Autodesk Inventor part; units mm, degrees
ref_plane "YZ Plane" through (0, 0, 0) normal (1, 0, 0) x (0, 1, 0)
ref_plane "XZ Plane" through (0, 0, 0) normal (0, 1, 0) x (-1, 0, 0)
ref_plane "XY Plane" through (0, 0, 0) normal (0, 0, 1) x (1, 0, 0)
sketch "Sketch1" plane through (0, 0, 0) normal (0, 0, 1) x (1, 0, 0)
  circle A0 centre (0, 0) radius 47.5 construction
  line L0 (-46.4354, 10) -> (-46.4354, -10) construction
  circle A1 centre (0, 0) radius 42.5 construction
  line L1 (-46.4354, 10) -> (-41.3068, 10)
  line L2 (-46.4354, -10) -> (-41.3068, -10)
  arc A2 (-46.4354, -10) -> (-46.4354, 10) centre (0, 0) ccw
  arc A3 (-41.3068, -10) -> (-41.3068, 10) centre (0, 0) ccw
  circle A4 centre (0, 0) radius 4.5
  circle A5 centre (0, 0) radius 6.5
  line L3 (4.2426, 1.5) -> (47.4763, 1.5)
  line L4 (4.2426, -1.5) -> (47.4763, -1.5)
  arc A6 (4.2426, -1.5) -> (4.2426, 1.5) centre (0, 0) ccw
  arc A7 (47.4763, -1.5) -> (47.4763, 1.5) centre (0, 0) ccw
  line L5 (-3.4204, 2.9242) -> (-25.0372, 40.3657)
  line L6 (-0.8223, 4.4242) -> (-22.4391, 41.8657)
  line L7 (-0.8223, -4.4242) -> (-22.4391, -41.8657)
  line L8 (-3.4204, -2.9242) -> (-25.0372, -40.3657)
  arc A8 (-0.8223, 4.4242) -> (-3.4204, 2.9242) centre (0, 0) ccw
  arc A9 (-3.4204, -2.9242) -> (-0.8223, -4.4242) centre (0, 0) ccw
  arc A10 (-22.4391, 41.8657) -> (-25.0372, 40.3657) centre (0, 0) ccw
  arc A11 (-25.0372, -40.3657) -> (-22.4391, -41.8657) centre (0, 0) ccw
  point P0 (-46.4354, 0)
  dimension "d0" = 95
  dimension "d1" = 20
  dimension "d2" = 5
  dimension "d5" = 9
  dimension "d7" = 3
  dimension "d10" = 360
  dimension "d17" = 13
extrude "Extrusion1" add sketch "Sketch1" along normal blind 15 contours A2 L5 A3 L1 | A2 L6 A3 L5 | A2 L3 A3 L6 | L5 A4 L8 A5 | A5 L6 A4 L5 | A2 L4 A3 L3 | A5 L3 A4 L6 | L8 A4 L7 A5 | A2 L7 A3 L4 | A5 L4 A4 L3 | L7 A4 L4 A5 | L8 A2 L2 A3 | A3 L7 A2 L8
extrude "Extrusion2" add sketch "Sketch1" along normal blind 5 contours A2 L6 A3 L5 | A3 L6 A5 L5 | A5 L6 A4 L5 | A2 L4 A3 L3 | A3 L4 A5 L3 | L8 A4 L7 A5 | A5 L7 A3 L8 | A5 L4 A4 L3 | A3 L7 A2 L8
sketch "Sketch3" plane through (0, 0, 15) normal (0, 0, 1) x (1, 0, 0)
  circle A0 centre (0, 0) radius 4.5
  circle A1 centre (0, 0) radius 6.5
  point P0 (0, 0)
extrude "Extrusion3" cut sketch "Sketch3" against normal blind 10
sketch "Sketch4" plane through (0, 0, 5) normal (0, 0, 1) x (1, 0, 0)
  arc A0 (6.3246, 1.5) -> (-1.8632, 6.2272) centre (0, 0) ccw
  line L0 (42.4735, 1.5) -> (6.3246, 1.5)
  circle A1 centre (0, 0) radius 6.5
  circle A2 centre (0, 0) radius 13.5
  point P0 (0, 0)
  dimension "d18" = 27
extrude "Extrusion4" cut sketch "Sketch4" against normal blind 3
properties part number "AA051" material "ABS Plastic"
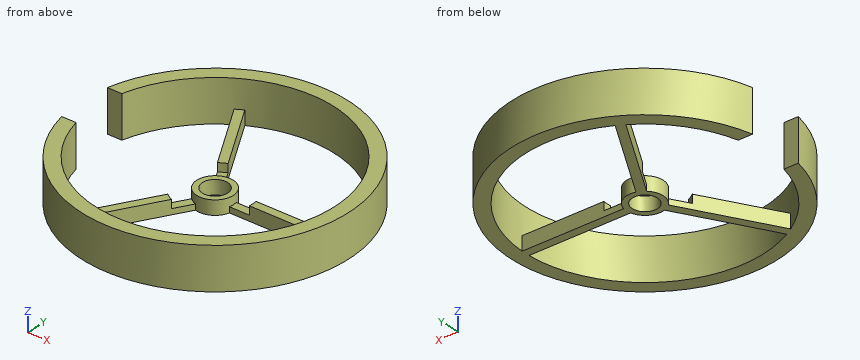
Geometry: final body of the model. Coordinates: model frame, mm. Round coordinates to 2 decimals unless told otherwise and drop trailing zeros. Write each loop counter-clockwise with the first axis right and the second up, starting at its lowest first coordinate (ties: lowest second). Pieces come first, ordered by that corner, then holes.
Item 1: Section query C-C (y = -14.5). Return loops of the section in (x, z).
Item 2: Section query B-B (y = 0). Return loops of the section in (x, z).
Item 3: Material intervals for L1, parallel to Y at x = 0, z = 3.05; L2, parallel to Y at x = 0, z = 9; L3, parallel to Y at x = 3, z = 3, sorted ascending.
Item 4: Section query D-D (x = 37). Return loops of the section in (y, z), plus the area to 3 significant figures.
Item 5: Pin query (flat end, axial travel): P1, Ø13.5, axis at x = -10, y = -22, coming from the +Z side; P2, Ø1, axis at x = -36.5, z = 10.5, coming from the -Y side; P3, Ø6, axis at x = 28, z = 11.5, coming from the +Y side. Return the tip coordinate at first contact, or that it passes through.
Item 6: Section query A-A (x = 0). Return loops of the section in (y, z).
Completed:
1. outline: (-45.23, 0) - (-39.95, 0) - (-39.95, 15) - (-45.23, 15) - close; (-10.1, 0) - (-6.64, 0) - (-6.64, 5) - (-10.1, 5) - close; (39.95, 0) - (45.23, 0) - (45.23, 15) - (39.95, 15) - close
2. outline: (-6.5, 0) - (-4.5, 0) - (-4.5, 5) - (-6.5, 5) - close; (4.5, 0) - (47.5, 0) - (47.5, 15) - (42.5, 15) - (42.5, 5) - (13.5, 5) - (13.5, 2) - (6.5, 2) - (6.5, 5) - (4.5, 5) - close
3. L1: y = -47.5 to -42.5, -6.5 to -4.5, 4.5 to 6.5, 42.5 to 47.5
3. L2: y = -47.5 to -42.5, 42.5 to 47.5
3. L3: y = -47.41 to -42.39, -5.77 to -3.35, 3.35 to 5.77, 42.39 to 47.41
4. outline: (-29.79, 0) - (-20.91, 0) - (-20.91, 15) - (-29.79, 15) - close; (-1.5, 0) - (1.5, 0) - (1.5, 5) - (-1.5, 5) - close; (20.91, 0) - (29.79, 0) - (29.79, 15) - (20.91, 15) - close
4. area: 281 mm2
5. P1: stops at z = 5
5. P2: stops at y = -30.99
5. P3: stops at y = 40.39
6. outline: (-47.5, 0) - (-42.5, 0) - (-42.5, 15) - (-47.5, 15) - close; (-6.5, 0) - (-4.5, 0) - (-4.5, 5) - (-6.5, 5) - close; (4.5, 0) - (6.5, 0) - (6.5, 5) - (4.5, 5) - close; (42.5, 0) - (47.5, 0) - (47.5, 15) - (42.5, 15) - close
